from build123d import *

# Parameters (mm, degrees)
SKETCH1_R           = 5
BOSS_EXTRUDE1_DEPTH = 1
SKETCH2_W           = 4.8
SKETCH2_H           = 4.8
BOSS_EXTRUDE2_DEPTH = 1.2
SKETCH3_W           = 1.5
SKETCH3_H           = 1
SKETCH3_W_2         = 0.75
BOSS_EXTRUDE3_DEPTH = 0.8


with BuildPart() as part:
    # Sketch1 → Boss-Extrude1 (new body)
    with BuildSketch(Plane.XY):
        Circle(SKETCH1_R)
    extrude(amount=BOSS_EXTRUDE1_DEPTH)

    # Sketch2 → Boss-Extrude2 (add)
    with BuildSketch(Plane.XY.offset(1)):
        Rectangle(SKETCH2_W, SKETCH2_H)
    extrude(amount=BOSS_EXTRUDE2_DEPTH)

    # Sketch3 → Boss-Extrude3 (add)
    with BuildSketch(Plane.XY.offset(1)):
        with Locations((0, -3.7)):
            Rectangle(SKETCH3_W, SKETCH3_H)
        with Locations((0.375, 3.7)):
            Rectangle(SKETCH3_W_2, SKETCH3_H)
        with Locations((-0.375, 3.7)):
            Rectangle(SKETCH3_W_2, SKETCH3_H)
    extrude(amount=BOSS_EXTRUDE3_DEPTH)


solid = part.part
The model under review builds one solid part; all positions refer to its coordinate system, in mm. A direction names the side the tool comes from. Round coordinates to 2 decimals unless told otherwise and drop trailing zeros. Write each loop counter-clockwise with the first axis right and the second up, starting at its lowest first coordinate (ties: lowest second). Pieces come first, ordered by that corner, then holes. Notation, with made-up numbers: M -26,63 L -6,63 A12 ccw -6,67 Z; hole C 56,-27 d9. An arc over 180 degrees is marked long. Use a Markdown table: item, result. Add a question column.
Q1. Insertion check: pin 1 (0.5 mm diameter, centred on x = 0.5, y = -3.5, fed in from +Z); pin 2 (6 mm diameter, centred on x = 3, y = -4, fed in from -Z); pin 3 (0.9 mm diameter, centred on x = 0, z = 1.5, fed in from -Y); pin 4 (0.9 mm diameter, centred on x = -0.5, z = 1.5, fed in from +Y). Each pin has a flat end and moves straight along its axis. Give the tip position at first contact, or say it passes through.
Q2. To check wall thickness, follow line 1 (Y direction, x = 0.25, z = 1.65); line 2 (Z direction, x = -3, y = 3); line 3 (X direction, y = 1.5, z = 1.55). State the ranges of each line that lie inside material, in increasing order.
Q3. Machinability: for faces 1 (the face through (0, -4, 1.8)), 2 (the face through (0, -2.4, 2)), 3 (the face through (0, 0, 2.2)), 4 (the face through (-2.4, 0, 2)), 5 (the face through (2.4, 0, 2)), which of the approach directions +Z, -Z, +X, -X, +Y, -Y give a long, thin tool a straight path to every point of the face, cutting with its end or side? Answer none if there is none.
Q4. We need section C-C, the plane y = -4. State the section outline as (x, z) points, plus the area to 3 significant figures.
Q5. The part is to be moulded in two halves that separate along Y. For faces 6 (the face through (0, 4, 1.8)), 7 (the face through (-1.08, -4.88, 0.49)), 8 (the face through (0, 2.4, 2)), say which applies: pulls with the +Y half, pulls with the -Y half, needs draft (parallel to the pull), parting line crosses it, or undercut.
Q6. We need section A-A, the plane y = 0. State the section outline as (x, z) points, plus the area to 3 significant figures.
Q7. We need section D-D, the plane z = 0.2. State the section outline as (x, y) points, plus the area to 3 significant figures.
Q8. We need section B-B, the plane x = 0. State the section outline as (y, z) points.
Findings below:
| question | item | result |
|---|---|---|
| 1 | pin 1 | stops at z = 1.8 |
| 1 | pin 2 | stops at z = 0 |
| 1 | pin 3 | stops at y = -4.2 |
| 1 | pin 4 | stops at y = 4.2 |
| 2 | line 1 | y = -4.2 to -3.2, -2.4 to 2.4, 3.2 to 4.2 |
| 2 | line 2 | z = 0 to 1 |
| 2 | line 3 | x = -2.4 to 2.4 |
| 3 | face 1 | +Z, +X, -X, -Y |
| 3 | face 2 | +Z, +X, -X |
| 3 | face 3 | +Z, +X, -X, +Y, -Y |
| 3 | face 4 | +Z, -X, +Y, -Y |
| 3 | face 5 | +Z, +X, +Y, -Y |
| 4 | outline | M -3,0 L 3,0 L 3,1 L 0.75,1 L 0.75,1.8 L -0.75,1.8 L -0.75,1 L -3,1 Z |
| 4 | area | 7.20 mm² |
| 5 | face 6 | needs draft |
| 5 | face 7 | parting line crosses it |
| 5 | face 8 | undercut |
| 6 | outline | M -5,0 L 5,0 L 5,1 L 2.4,1 L 2.4,2.2 L -2.4,2.2 L -2.4,1 L -5,1 Z |
| 6 | area | 15.8 mm² |
| 7 | outline | C 0,0 d10 |
| 7 | area | 78.5 mm² |
| 8 | outline | M -5,0 L 5,0 L 5,1 L 4.2,1 L 4.2,1.8 L 3.2,1.8 L 3.2,1 L 2.4,1 L 2.4,2.2 L -2.4,2.2 L -2.4,1 L -3.2,1 L -3.2,1.8 L -4.2,1.8 L -4.2,1 L -5,1 Z |
